Could you check a few things on this drawing? It's one solid part, dimensions in mm from its lowest x, y, z. A direction names the side the tool comes from. Round coordinates to 2 decimals unless told otherwise and drop trailing zeros. Order: outer loops, then holes, each group sorted by start corner. A loop starts at its lowest first (then second) coordinate and runs counter-clockwise, first axis right, second up.
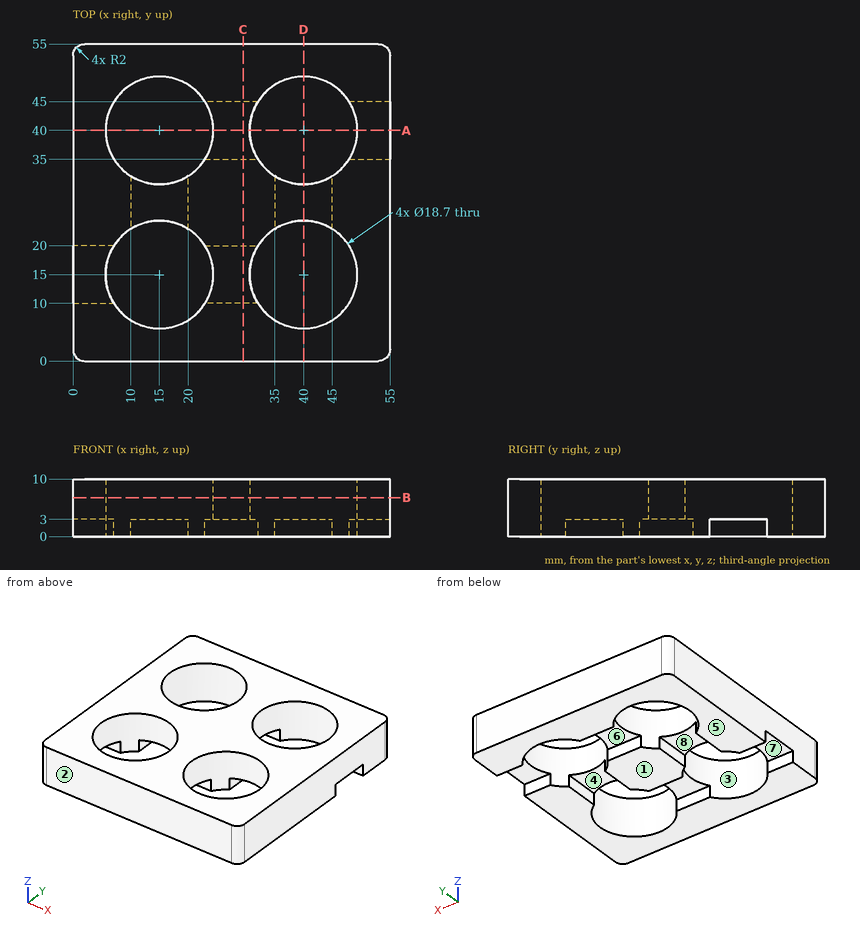
(1) Please list where these lines run through material, in increasing order: probe 1 along X at (y, z) = (15, 4); probe 2 along Y at (x, z) = (39.5, 8.5); probe 3 along Y at (x, z) = (15.5, 1.25).
(2) On a 3-axis mill with a long thin cutter (end or side, diameter ignored), from which of +Z, -Z, +X, -X, +Y, -Y can I reach the whole of each face in a straight line? I mean the marked faces 5, 6, 7 and 8. Say none if no direction works.
(3) I want a section at B-B, the plane z = 6.75. List the corners of the cut face in (x, y) for me, plus the area to 3 significant figures.
(4) I'm going to push a flat-ended pin straight in: pin 1 Ø8 at (x, y) = (5, 15) entering from -Z. Where does the tip first touch, or does it pass through?
(5) If we mould it in two halves opening along Y, with no side actions, what happens to the marked faces 1, 2, 3 and 4? For each: pulls with the +Y half, pulls with the -Y half, needs draft (parallel to the pull), parting line crosses it, or undercut.
(6) I want a section at A-A, the plane y = 40. List the corners of the cut face in (x, z) for me, plus the area to 3 significant figures.
(7) I want a section at D-D, the plane x = 40. List the corners of the cut face in (y, z) for me.
(8) I want a section at C-C, the plane x = 29.5. List the corners of the cut face in (y, z) for me, plus the area to 3 significant figures.
Ans:
1. probe 1: x = 0 to 5.65, 24.35 to 30.65, 49.35 to 55
1. probe 2: y = 0 to 5.66, 24.34 to 30.66, 49.34 to 55
1. probe 3: y = 0 to 5.66, 49.34 to 55
2. face 5: -Z, +X, -X, +Y, -Y
2. face 6: -Z, +X
2. face 7: -Z, -X
2. face 8: -Z
3. outline: (0, 2) arc R2 ccw to (2, 0) - (53, 0) arc R2 ccw to (55, 2) - (55, 53) arc R2 ccw to (53, 55) - (2, 55) arc R2 ccw to (0, 53) - close; hole circle Ø18.7 at (15, 15); hole circle Ø18.7 at (15, 40); hole circle Ø18.7 at (40, 15); hole circle Ø18.7 at (40, 40)
3. area: 1,920 mm2
4. pin 1: stops at z = 3
5. face 1: needs draft
5. face 2: pulls with the -Y half
5. face 3: undercut
5. face 4: undercut
6. outline: (0, 0) - (5.65, 0) - (5.65, 10) - (0, 10) - close; (24.35, 3) - (30.65, 3) - (30.65, 10) - (24.35, 10) - close; (49.35, 3) - (55, 3) - (55, 10) - (49.35, 10) - close
6. area: 140 mm2
7. outline: (0, 0) - (5.65, 0) - (5.65, 10) - (0, 10) - close; (24.35, 3) - (30.65, 3) - (30.65, 10) - (24.35, 10) - close; (49.35, 0) - (55, 0) - (55, 10) - (49.35, 10) - close
8. outline: (0, 0) - (10, 0) - (10, 3) - (20, 3) - (20, 0) - (35, 0) - (35, 3) - (45, 3) - (45, 0) - (55, 0) - (55, 10) - (0, 10) - close
8. area: 490 mm2
